Verification items for the finished model (mm, model axes). A direction names the side the tool comes from. Round coordinates to 2 decimals unless told otherwise and drop trailing zeros. Order: outer loops, then holes, each group sorted by start corner. A loop starts at its lowest first (then second) coordinate and runs counter-clockwise, first axis right, second up. Notation, with made-up numbers: M -25,23.25 L 4,23.25 A25 ccw 4,52.25 Z; hole C 52.25,30.25 d6. An arc over 180 degrees is marked long. Use CSV: the item, a comma, the result in double quotes. Start each with the question number.
Q1. Sectioned sample at C-C (x = -0.2). Enter the section's corners in (y, z).
Q2. Sectioned sample at B-B (z = 0). Enter the section's corners in (x, y).
Q3. Sectioned sample at D-D (x = 1.1). Enter the section's corners in (y, z), and give its area (3 significant figures).
Q4. Set-up check for faces 1 (the face through (0.91, -0.49, -0.06)), 2 (the face through (1.863, -3.465, 0.24)), 3 (the face through (-1, -6, 0)): record each of +Z, -Z, +X, -X, +Y, -Y from which the full face is reachable in a straight line by a thin tool's end or side.
Q5. Sectioned sample at A-A (x = -2.65). Enter the section's corners in (y, z), and give its area (3 significant figures).
Q6. Mould release check, pull along Z, two halves, no side actions. Record for faces 4 (the face through (-1, 1, -1)), 5 (the face through (-1.17, 0.99, 2.42)), 6 (the face through (-1.633, 1.493, 0.341)), 7 (the face through (1, 2, 0)): +Z half, -Z half, draft (parallel to the pull), parting line (faces both ways), or undercut.
Q7. Scan lines: line 1 (Y direction, x = 0.8, z = 0.85); line 2 (Z direction, x = -0.55, y = -2.5); line 3 (Y direction, x = 0.75, z = 1.75). Record each from-to range of solid material in increasing order.
```python
from build123d import *

# Parameters (mm, degrees)
SKETCH1_R           = 3
SKETCH1_R_2         = 1.4
BOSS_EXTRUDE1_DEPTH = 2
SKETCH1_3_R         = 1.4
BOSS_EXTRUDE2_DEPTH = 1
SKETCH5_R           = 1.5
BOSS_EXTRUDE3_DEPTH = 1
SKETCH6_R           = 2.5
BOSS_EXTRUDE4_DEPTH = 5


with BuildPart() as part:
    # Sketch1 → Boss-Extrude1 (new body)
    with BuildSketch(Plane(origin=(0, 0, 0), x_dir=(1, 0, 0), z_dir=(0, 1, 0))):
        with Locations((-0.522013312, 0.511138034)):
            Circle(SKETCH1_R)
        with Locations((-0.522013312, 0.511138034)):
            Circle(SKETCH1_R_2, mode=Mode.SUBTRACT)
    extrude(amount=BOSS_EXTRUDE1_DEPTH)

    # Sketch1<3> → Boss-Extrude2 (add)
    with BuildSketch(Plane(origin=(0, 0, 0), x_dir=(1, 0, 0), z_dir=(0, 1, 0))):
        with Locations((-0.522013312, 0.511138034)):
            Circle(SKETCH1_3_R)
    extrude(amount=BOSS_EXTRUDE2_DEPTH)

    # Sketch5 → Boss-Extrude3 (add)
    with BuildSketch(Plane.XZ):
        with Locations((-0.522013312, -0.511138034)):
            Circle(SKETCH5_R)
    extrude(amount=BOSS_EXTRUDE3_DEPTH)

    # Sketch6 → Boss-Extrude4 (add)
    with BuildSketch(Plane.XZ.offset(1)):
        with Locations((-0.522013312, -0.511138034)):
            Circle(SKETCH6_R)
    extrude(amount=BOSS_EXTRUDE4_DEPTH)


solid = part.part
```
Verdict:
1,outline,"M -6,-2.99 L -1,-2.99 L -1,-1.98 L 0,-1.98 L 0,-3.49 L 2,-3.49 L 2,-1.87 L 1,-1.87 L 1,0.85 L 2,0.85 L 2,2.47 L 0,2.47 L 0,0.95 L -1,0.95 L -1,1.97 L -6,1.97 Z"
2,outline,"M -3.48,0 L -1.93,0 L -1.93,-1 L -2.97,-1 L -2.97,-6 L 1.93,-6 L 1.93,-1 L 0.89,-1 L 0.89,0 L 2.43,0 L 2.43,2 L 0.78,2 L 0.78,1 L -1.83,1 L -1.83,2 L -3.48,2 Z"
3,outline,"M -6,-2.41 L -1,-2.41 L -1,1.39 L -6,1.39 Z; M 0,-3.03 L 2,-3.03 L 2,2.01 L 0,2.01 Z"
3,area,"29.1 mm²"
4,face 1,"none"
4,face 2,"-Y"
4,face 3,"+Z, -Z, +X, -X, -Y"
5,outline,"M -6,-1.82 L -1,-1.82 L -1,0.8 L -6,0.8 Z; M 0,-2.63 L 2,-2.63 L 2,1.6 L 0,1.6 Z"
5,area,"21.6 mm²"
6,face 4,"undercut"
6,face 5,"parting line"
6,face 6,"undercut"
6,face 7,"draft"
7,line 1,"y = -6 to -1, 0 to 2"
7,line 2,"z = -3.01 to 1.99"
7,line 3,"y = 0 to 2"
